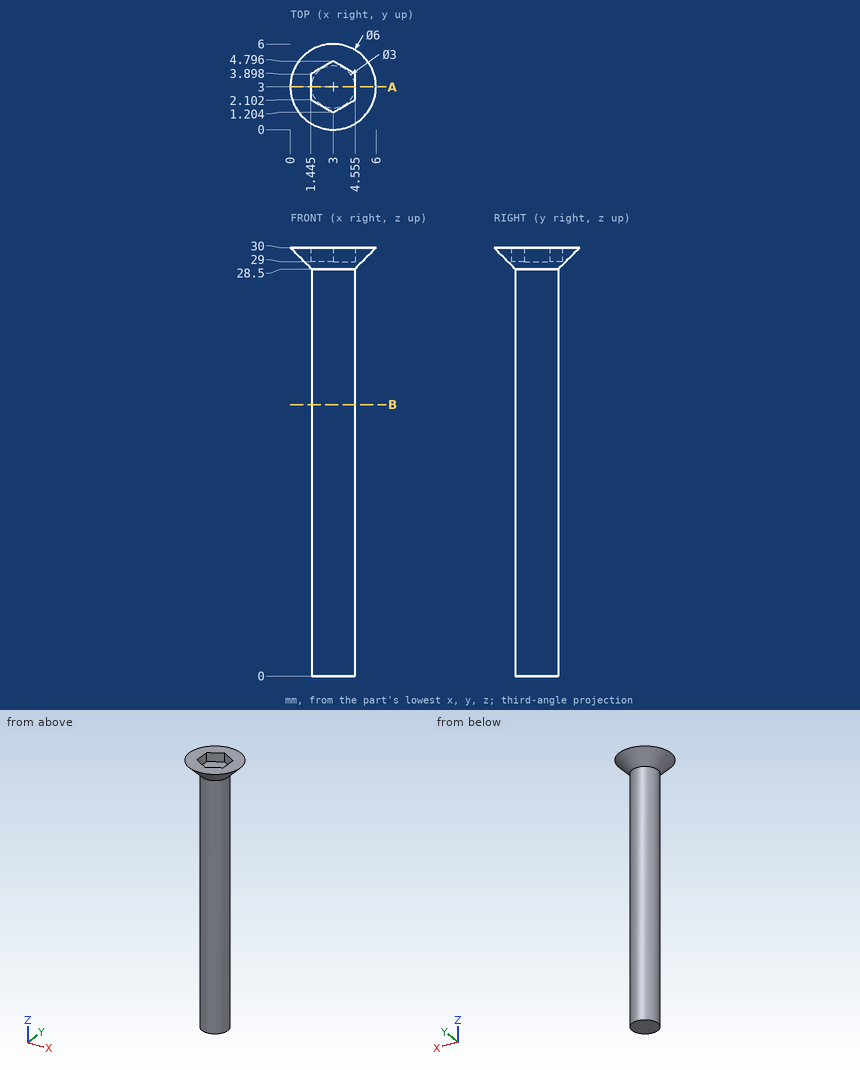
Design review of the part shown in the three views and the two pictorial views. Dimensions are in mm from the part's minimum x, y and z. Round coordinates to 2 decimals unless told otherwise and drop trailing zeros. Loops run counter-clockwise (first coordinate to the right, second up) from the corner with the lowest first, then second, coordinate; pieces in that order, holes last.
Q1. Insertion check: pin 1 Ø0.8 at (y, z) = (3, 29.5) entering from -X; pin 2 Ø0.5 at (y, z) = (3.5, 29.5) entering from +X; pin 3 Ø1 at (y, z) = (1.5, 23.5) entering from -X. Each pin has a flat end and moves straight along its axis. Give the tip position at first contact, or say it passes through.
Result sheet:
pin 1: stops at x = 0.1
pin 2: stops at x = 5.71
pin 3: stops at x = 1.88
Q2. To check wall thickness, follow line 1 along Z through (x, y) = (3.3, 1.7); line 2 along X through (y, z) = (4.2, 11.75); line 3 along Y through (x, z) = (2.95, 19.5). State the ranges of each line that lie inside material, in increasing order.
Result sheet:
line 1: z = 0 to 29
line 2: x = 2.1 to 3.9
line 3: y = 1.5 to 4.5
Q3. Add section B-B on z = 19. Write out the cut boundary in (x, y).
Result sheet:
outline: circle Ø3 at (3, 3)
Q4. Add section A-A on y = 3. Write out the cut boundary in (x, z) (1 decimal).
Result sheet:
outline: (0, 30) - (1.5, 28.5) - (1.5, 0) - (4.5, 0) - (4.5, 28.5) - (6, 30) - (4.6, 30) - (4.6, 29) - (1.4, 29) - (1.4, 30) - close
